Can you work these out from the model? Positions are in its coordinate system, mm. A direction names the side the tool comes from. Give positions to 0.01 mm unless a question says otherwise; leave off trailing zeros. Order: outer loops, then holes, each group sorted by start corner. A loop starts at its lowest first (then second) coordinate and runs counter-clockwise, first axis right, second up. Notation, with made-up numbers: M -12,33.25 L -7,33.25 A10 ccw -7,39.25 Z; hole C 87.25,3 d7. An arc over 180 degrees is marked long. Use one line per item in the form item = value. Start each with the question number.
1. I need wall thicknesses on L1, parallel to X at y = 37, z = -2.25; L2, parallel to X at y = 21, z = -1.75; L3, parallel to Y at x = -7.25, z = -2. Which ranges of each line are inside material? Lowest first, please.
2. For faces 1 (the face through (2.442, 33.375, 5.889)), 2 (the face through (0, 36.5, 0)), which set-ups out of +Z, -Z, +X, -X, +Y, -Y let a thin tool reach every point of the face, with its end or its side?
3. We'd pull the mould along X, two halves only. Please class faces 3 (the face through (-6, 39, 0)), 4 (the face through (-1.802, 19.689, 5.723)), 5 (the face through (-1.25, 38, 0)): +X half, -X half, draft (parallel to the pull), parting line (faces both ways), or undercut.
4. Will these pins go through, and if not, where does the flat tip stop? P1, Ø1.3, axis at x = 0.5, z = -2, coming from the +Y side; P2, Ø5, axis at x = 7.5, z = -1.5, coming from the -Y side; P3, Ø2, axis at y = 37.5, z = -2, coming from the -X side.
5. I want a section at B-B, the plane y = 5.5. List the corners of the cut face in (x, z) for me, and give its area (3 significant figures).
6. I want a section at A-A, the plane y = 37. List the corners of the cut face in (x, z) for me, and give its area (3 significant figures).
```python
from build123d import *

# Parameters (mm, degrees)
CUT_EXTRUDE1_DEPTH      = 43.532340636
CUT_EXTRUDE1_DEPTH_BACK = 43.532340636
SKETCH2_W               = 2.5
SKETCH2_H               = 2.5


with BuildPart() as part:
    # Sketch1 → Revolve1 (revolve)
    with BuildSketch(Plane(origin=(0, 0, 0), x_dir=(0, 0, -1), z_dir=(1, 0, 0)), mode=Mode.PRIVATE) as revolve1_sk:
        Polygon((0, 0), (6, 6), (6, 33), (12, 39), (0, 39), align=None)
    revolve(revolve1_sk.sketch.rotate(Axis((0, 39, 0), (0, -1, 0)), 180), axis=Axis((0, 39, 0), (0, -1, 0)))

    # Sketch2 → Cut-Extrude1 (cut, two sides: drawn at the far end of the back side and taken through both)
    with BuildSketch(Plane.XY.offset(-CUT_EXTRUDE1_DEPTH_BACK)):
        with Locations((0, 37.75)):
            Rectangle(SKETCH2_W, SKETCH2_H)
    extrude(amount=CUT_EXTRUDE1_DEPTH + CUT_EXTRUDE1_DEPTH_BACK, mode=Mode.SUBTRACT)


solid = part.part
```
Check result:
q1.L1 = -9.74 to -1.25, 1.25 to 9.74
q1.L2 = -5.74 to 5.74
q1.L3 = 34.52 to 39
q2.face_1 = -Y
q2.face_2 = +Z, -Z, +Y
q3.face_3 = draft
q3.face_4 = parting line
q3.face_5 = undercut
q4.P1 = 36.5
q4.P2 = 5.15
q4.P3 = -11.34
q5.outline = C 0,0 d11
q5.area = 95.0 mm2
q6.outline = M -1.25,-9.92 L -1.25,9.92 A10 ccw Z; M 1.25,-9.92 A10 ccw 1.25,9.92 Z
q6.area = 264 mm2
